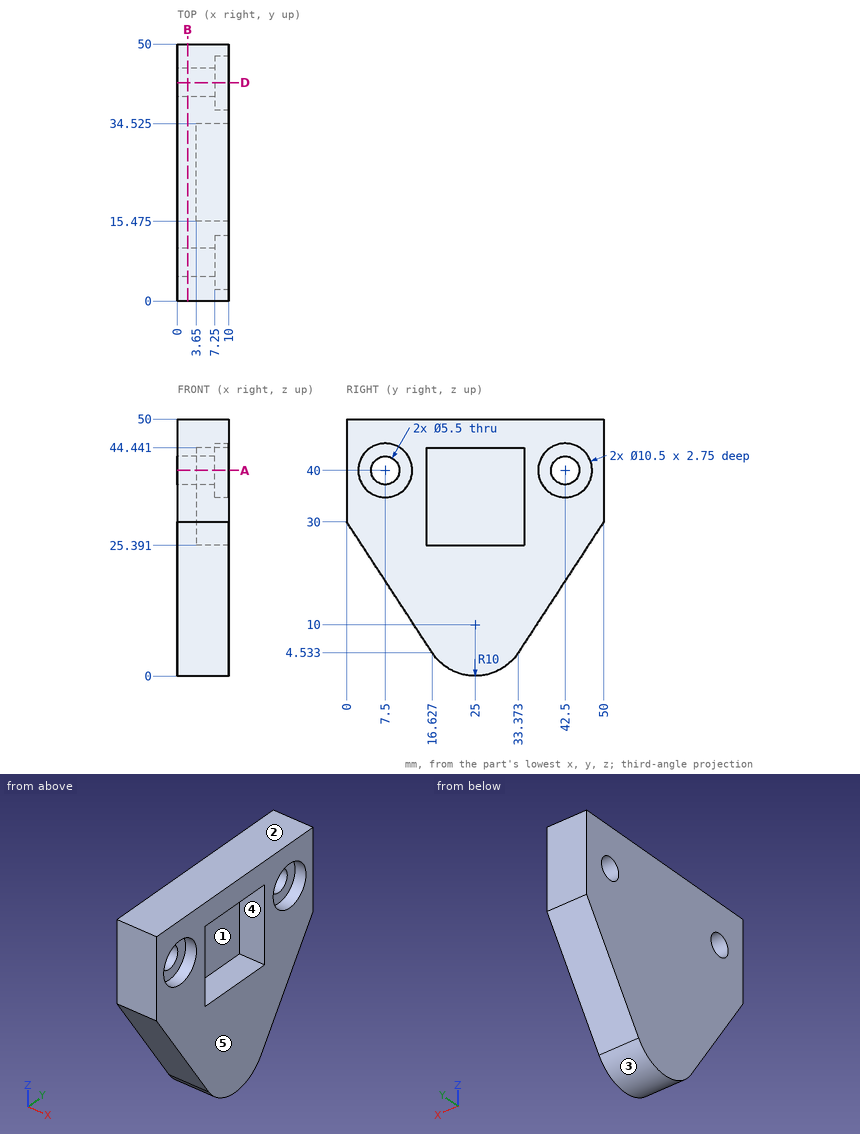
Input: dimensioned drawing with shaded views. Units: mm. Origin: part minimum x, y, z. A direction names the side the tool comes from. Give positions to 0.01 mm unless a question says otherwise; leave off trailing zeros. Write each loop counter-clockwise with the first axis right and the second up, starting at its lowest first coordinate (ties: lowest second). Pieces come first, ordered by that corner, then holes.
1. Section query A-A, the plane z = 40. Count the separate pieces of the cut face and the enclosed holes in it.
2. Section query B-B, the plane x = 2. Return loops of the section in (y, z).
3. Draft query along Z for the marked faces 1, 2 and 3. Return one class per face: released by +Z, released by -Z, zero draft, split by the parting line, or undercut.
4. Section query D-D, the plane y = 42.5. Return loops of the section in (x, z), then the cut area to 3 significant figures.
5. Line query: probe 1 along Y at (x, z) = (3.25, 40); probe 2 along Z at (x, y) = (5, 25.5); probe 3 along Y at (x, z) = (7, 33) (1 decimal). Output: solid intervals per line, ascending.
6. Reachability of the marked faces 4 and 5 from +Z, -Z, +X, -X, +Y, -Y: full face, straight path, thin tool, end or side. Return the list, or none.
7. Pin query (flat end, axial travel): P1, Ø3.5, axis at y = 42.5, z = 40, coming from the -X side; P2, Ø3, axis at x = 6, y = 22.5, coming from the -Z side; P3, Ø2, axis at x = 4, y = 30.5, coming from the -Z side; P4, Ø8.5, axis at y = 42.5, z = 40, coming from the +X side. Return the tip coordinate at first contact, or that it passes through.
Computed:
1. separate pieces: 3
1. enclosed holes: 0
2. outline: (0, 30) - (16.63, 4.53) arc R10 ccw to (33.37, 4.53) - (50, 30) - (50, 50) - (0, 50) - close; hole circle Ø5.5 at (7.5, 40); hole circle Ø5.5 at (42.5, 40)
3. face 1: undercut
3. face 2: released by +Z
3. face 3: released by -Z
4. outline: (0, 18.51) - (10, 18.51) - (10, 34.75) - (7.25, 34.75) - (7.25, 37.25) - (0, 37.25) - close; (0, 42.75) - (7.25, 42.75) - (7.25, 45.25) - (10, 45.25) - (10, 50) - (0, 50) - close
4. area: 246 mm2
5. probe 1: y = 0 to 4.75, 10.25 to 39.75, 45.25 to 50
5. probe 2: z = 0.01 to 25.39, 44.44 to 50
5. probe 3: y = 0 to 15.5, 34.5 to 50
6. face 4: +X
6. face 5: +Z, -Z, +X, +Y, -Y
7. P1: passes through
7. P2: stops at z = 0.05
7. P3: stops at z = 1.07
7. P4: stops at x = 7.25
